from build123d import *

# Parameters (mm, degrees)
F1_DEPTH = 60
F2_DEPTH = 9
F3_DEPTH = 25
F5_R     = 10


with BuildPart() as f1:
    # F0 (on Front) → F1 (new body, symmetric)
    with BuildSketch(Plane.XZ):
        Polygon((0, 20), (0, 0), (80, 0), (80, 20), (60, 20), align=None)
    extrude(amount=F1_DEPTH, both=True)

    # F0 (on Front) → F2 (join, symmetric)
    with BuildSketch(Plane.XZ):
        with BuildLine():
            ThreePointArc((95, 70), (41.322724, 56.736825), (0, 20))
            Line((0, 20), (60, 20))
            Line((60, 20), (60, 35))
            ThreePointArc((60, 35), (70.251263, 59.748737), (95, 70))
        make_face()
    extrude(amount=F2_DEPTH, both=True)

    # F0 (on Front) → F3 (join, symmetric)
    with BuildSketch(Plane.XZ):
        with BuildLine():
            Line((60, 20), (80, 20))
            Line((80, 20), (80, 35))
            ThreePointArc((80, 35), (84.393398, 45.606602), (95, 50))
            Line((95, 50), (125, 50))
            Line((125, 50), (125, 70))
            Line((125, 70), (95, 70))
            ThreePointArc((95, 70), (70.251263, 59.748737), (60, 35))
            Line((60, 35), (60, 20))
        make_face()
    extrude(amount=F3_DEPTH, both=True)

    # F0 (on Front) → F4 (revolve)
    with BuildSketch(Plane.XZ):
        Polygon((125, 75), (125, 70), (125, 50), (125, 45), (150, 45), (150, 75), align=None)
    revolve(axis=Axis((125, 0, 60), (0, 0, 1)))

    # F5
    f5_edges = [f1.edges().sort_by_distance(p)[0] for p in [
        (0, -60, 10),
        (80, -60, 10),
        (0, 60, 10),
        (80, 60, 10),
    ]]
    fillet(f5_edges, radius=F5_R)


solid = f1.part
Could you check a few things on this model? Use its own coordinates, in mm. A direction names the side the tool comes from. Give positions to 0.01 mm unless a question says otherwise; leave off trailing zeros. Loops run counter-clockwise (first coordinate to the right, second up) from the corner with the lowest first, then second, coordinate; pieces in that order, holes last. Notation, with made-up numbers: M 16,34.25 L 71,34.25 A16 cw 71,51.25 Z; hole C 66,-27 d2. An arc over 180 degrees is marked long. Answer as a JSON object with one key per item and string values.
Q1. Suppose I cut it at B-B, the plane x = 14. List the corners of the cut face in (y, z) for me, plus the area to 3 significant figures.
Values found:
{"outline": "M -60,0 L 60,0 L 60,20 L 9,20 L 9,36.74 L -9,36.74 L -9,20 L -60,20 Z", "area": "2,700 mm²"}
Q2. For faces 1 (the flat face through (125, 0, 45)), 2 (the cylindrical face through (70.525, 16.888, 60.019)), 3 (the flat face through (60, -17, 28)), which set-ups out of +Z, -Z, +X, -X, +Y, -Y let a thin tool reach every point of the face, with its end or its side?
Values found:
{"face 1": "-Z, +X, +Y, -Y", "face 2": "+Z, -X, +Y", "face 3": "+Z, -X, -Y"}
Q3. Suppose I cut it at C-C, the plane y = -17. List the corners of the cut face in (x, z) for me.
Values found:
{"outline": "M 0,0 L 80,0 L 80,35 A15 cw 95,50 L 106.67,50 L 106.67,45 L 143.33,45 L 143.33,75 L 106.67,75 L 106.67,70 L 95,70 A35 ccw 60,35 L 60,20 L 0,20 Z"}
Q4. If we mould it in two halves opening along X, with no side actions, what happens to faces 4 (the cylindrical face through (77.15, -56.99, 10.14)), 5 (the flat face through (100, 4, 70)), 6 (the flat face through (99.9, -2, 50))? For each: pulls with the +X half, pulls with the -X half, needs draft (parallel to the pull), parting line crosses it, or undercut.
Values found:
{"face 4": "pulls with the +X half", "face 5": "needs draft", "face 6": "undercut"}
Q5. For P1, Ø8, axis at y = 5.5, z = 50.5, coming from the -X side; P2, Ø10.5, axis at y = 21.5, z = 10, coming from the +X side; P3, Ø5, axis at x = 83, z = 53, coming from the -Y side, each with a flat end and sliding along its axis, tell me the tip position at first contact or that it passes through.
Values found:
{"P1": "stops at x = 25.25", "P2": "stops at x = 80", "P3": "stops at y = -25"}
Q6. Suppose I cut it at D-D, the plane x = 92. List the corners of the cut face in (y, z) for me.
Values found:
{"outline": "M -25,49.7 L 25,49.7 L 25,69.87 L 9,69.87 L 9,69.96 L -9,69.96 L -9,69.87 L -25,69.87 Z"}
Q7. Suppose I cut it at A-A, the plane y = 0. List the corners of the cut face in (x, z) for me.
Values found:
{"outline": "M 0,0 L 80,0 L 80,35 A15 cw 95,50 L 100,50 L 100,45 L 150,45 L 150,75 L 100,75 L 100,70 L 95,70 A115.25 ccw 0,20 Z"}
Q8. If I drill on probe 1 along Y at (x, z) = (55, 28); probe 2 along X at (y, z) = (-8.5, 11.5); probe 3 along Z at (x, y) = (29, 29.5), over which ranges is the centre line in solid material (lowest first)? Write a range as [from, to].
Values found:
{"probe 1": "y = [-9, 9]", "probe 2": "x = [0, 80]", "probe 3": "z = [0, 20]"}
